from build123d import *
from build123d.topology import SkipClean

# Parameters (mm, degrees)
BOSS_EXTRUDE1_START = -0.3
SKETCH3_R           = 1.4
BOSS_EXTRUDE1_DEPTH = 0.3
SKETCH4_R           = 0.349337209
SKETCH4_R_2         = 0.249337209
CUT_EXTRUDE6_START  = -0.7
SKETCH8_R           = 0.249337209
CUT_EXTRUDE6_DEPTH  = 0.7
CUT_EXTRUDE7_START  = -0.3
SKETCH4_5_R         = 0.249337209
CUT_EXTRUDE7_DEPTH  = 0.3


with BuildPart() as part:
    # Sketch2 → Revolve1 (revolve)
    with BuildSketch(Plane(origin=(0, 0, 0), x_dir=(0, 0, -1), z_dir=(1, 0, 0))):
        Polygon((0, 0), (2.5, 0), (2.5, 3), (1.9, 3), (1.9, 5), (1.4, 5), (1.4, 2.5), (2, 2.5), (2, 0.5), (0, 0.5), align=None)
    revolve(axis=Axis((0, 0, 0), (0, 1, 0)))

    # Sketch3 → Boss-Extrude1 (add)
    with BuildSketch(Plane(origin=(0, 4.5, 0), x_dir=(1, 0, 0), z_dir=(0, 1, 0)).offset(BOSS_EXTRUDE1_START)):
        with Locations(Location((0, 0, 0), (0, 0, 90))):
            Circle(SKETCH3_R)
    extrude(amount=BOSS_EXTRUDE1_DEPTH)

    # Sweep2: sweep along a path in Sketch5
    with BuildLine(Plane.XY) as sweep2_path:
        Line((0.6, 4.5), (0.6, 2))
        Line((0.6, 2), (1.3, 2))
        Line((1.3, 2), (1.3, 0.5))
    # Sketch4 → Sweep2 (sweep)
    with BuildSketch(Plane(origin=(0, 4.5, 0), x_dir=(1, 0, 0), z_dir=(0, 1, 0))):
        with Locations((0.6, 0)):
            Circle(SKETCH4_R)
        with Locations((0.6, 0)):
            Circle(SKETCH4_R_2, mode=Mode.SUBTRACT)
    sweep2 = sweep(path=sweep2_path.line, transition=Transition.RIGHT)

    # Sketch8 → Cut-Extrude6 (cut)
    with BuildSketch(Plane(origin=(0, 0.5, 0), x_dir=(1, 0, 0), z_dir=(0, 1, 0)).offset(CUT_EXTRUDE6_START)):
        with Locations((1.3, 0)):
            Circle(SKETCH8_R)
    cut_extrude6 = extrude(amount=CUT_EXTRUDE6_DEPTH, mode=Mode.SUBTRACT)

    # Sketch4_5 → Cut-Extrude7 (cut)
    with SkipClean():  # the faces are left unmerged after this step: merging them gives an invalid solid
        with BuildSketch(Plane(origin=(0, 4.5, 0), x_dir=(1, 0, 0), z_dir=(0, 1, 0)).offset(CUT_EXTRUDE7_START)):
            with Locations(Location((0.6, 0, 0), (0, 0, 270))):
                Circle(SKETCH4_5_R)
        cut_extrude7 = extrude(amount=CUT_EXTRUDE7_DEPTH, mode=Mode.SUBTRACT)
    add(part.part.scale(1), mode=Mode.REPLACE)  # the faces are merged on a copy

    # Mirror1: Sweep2, Cut-Extrude6, Cut-Extrude7 across plane
    with SkipClean():  # the faces are left unmerged after this step: merging them gives an invalid solid
        add(sweep2.mirror(Plane(origin=(0, 0, 0), x_dir=(0, 0, 1), z_dir=(1, 0, 0))))
        add(cut_extrude6.mirror(Plane(origin=(0, 0, 0), x_dir=(0, 0, 1), z_dir=(1, 0, 0))), mode=Mode.SUBTRACT)
        add(cut_extrude7.mirror(Plane(origin=(0, 0, 0), x_dir=(0, 0, 1), z_dir=(1, 0, 0))), mode=Mode.SUBTRACT)


solid = part.part
Geometry check sheet. Reference: the model listing, model coordinates, mm. A direction names the side the tool comes from. Round coordinates to 2 decimals unless told otherwise and drop trailing zeros. Write each loop counter-clockwise with the first axis right and the second up, starting at its lowest first coordinate (ties: lowest second). Pieces come first, ordered by that corner, then holes. Notation, with made-up numbers: (-9.5, -15.75) - (41.5, -15.75) arc R12 cw to (41.5, -2.75) - close; hole circle Ø11 at (15.5, -25.5). An arc over 180 degrees is marked (long way). One line per item, written item: value.
1. Depth check by flat-ended pin: pin 1 Ø1 at (y, z) = (4.5, -0.5) entering from +X; pin 2 Ø2 at (y, z) = (3.5, 1.5) entering from -X. Enter the tip coordinate at first touch or a pass-through.
The answers:
pin 1: stops at x = 1.9
pin 2: stops at x = -2.42
2. Scan lines: L1, parallel to Y at x = -0.4, z = -1.6; L2, parallel to X at y = 0.45, z = 0; L3, parallel to X at y = 4.95, z = 0. Record each from-to range of solid material in increasing order.
The answers:
L1: y = 0 to 0.5, 2.5 to 5
L2: x = -2.5 to -1.55, -1.05 to 1.05, 1.55 to 2.5
L3: x = -1.9 to -1.4, 1.4 to 1.9
3. Cross-section at A-A on y = 2. Record the boundary of the cut face in (x, z), and give its area (3 significant figures).
The answers:
outline: circle Ø5 at (0, 0); (-1.3, -0.35) - (-0.6, -0.35) arc R0.35 ccw to (-0.6, 0.35) - (-1.3, 0.35) arc R0.35 ccw to start; (0.6, -0.35) - (1.3, -0.35) arc R0.35 ccw to (1.3, 0.35) - (0.6, 0.35) arc R0.35 ccw to start; hole circle Ø4 at (0, 0); hole (-1.3, -0.25) - (-0.6, -0.25) arc R0.25 ccw to (-0.6, 0.25) - (-1.3, 0.25) arc R0.25 ccw to start; hole (0.6, -0.25) - (1.3, -0.25) arc R0.25 ccw to (1.3, 0.25) - (0.6, 0.25) arc R0.25 ccw to start
area: 7.72 mm^2
4. Cross-section at B-B on z = -1.6. Record the boundary of the cut face in (x, y).
The answers:
outline: (-1.92, 0) - (1.92, 0) - (1.92, 3) - (1.02, 3) - (1.02, 5) - (-1.02, 5) - (-1.02, 3) - (-1.92, 3) - close; hole (-1.2, 0.5) - (1.2, 0.5) - (1.2, 2.5) - (-1.2, 2.5) - close
5. Set-up check for faces 1 (the face through (0, 4.2, 0)), 2 (the face through (0, 0, 0)), 3 (the face through (0, 4.5, 0)): record each of +Z, -Z, +X, -X, +Y, -Y from which the full face is reachable in a straight line by a thin tool's end or side.
The answers:
face 1: none
face 2: +Z, -Z, +X, -X, -Y
face 3: +Y
6. Cross-section at C-C on y = 2.8. Record the boundary of the cut face in (x, z).
The answers:
outline: circle Ø5 at (0, 0); circle Ø0.7 at (-0.6, 0); circle Ø0.7 at (0.6, 0); hole circle Ø2.8 at (0, 0); hole circle Ø0.5 at (-0.6, 0); hole circle Ø0.5 at (0.6, 0)
7. Cross-section at D-D on x = 1.3. Record the boundary of the cut face in (y, z).
The answers:
outline: (0, -2.14) - (3, -2.14) - (3, -1.39) - (5, -1.39) - (5, -0.52) - (4.5, -0.52) - (4.5, 0.52) - (5, 0.52) - (5, 1.39) - (3, 1.39) - (3, 2.14) - (0, 2.14) - (0, 0.25) - (2, 0.25) arc R0.25 cw to (2, -0.25) - (0, -0.25) - close; hole (0.5, -1.52) - (2.5, -1.52) - (2.5, -0.52) - (4.2, -0.52) - (4.2, 0.52) - (2.5, 0.52) - (2.5, 1.52) - (0.5, 1.52) - (0.5, 0.35) - (2, 0.35) arc R0.35 cw to (2, -0.35) - (0.5, -0.35) - close
8. Mould release check, pull along X, two halves, no side actions. Record for faces 4 (the face through (1.3, 2.5, 0.9)), 5 (the face through (2.44, 1.52, 0.54)), 6 (the face through (-1, 3, -2)): released by +X, released by -X, zero draft, split by the parting line, or undercut.
The answers:
face 4: undercut
face 5: split by the parting line
face 6: zero draft
